Check sheet for the modelled part. Datum: model origin and axes. Units: mm. Face numbers are marked on the shaded views. A direction names the side the tool comes from. Coordinates: 2 decimals unless noted, no trailing zeros. Loops run counter-clockwise (first coordinate to the right, second up) from the corner with the lowest first, then second, coordinate; pieces in that order, holes last. Notation, with made-up numbers: (-7.75, 42) -> (20.25, 42) arc R17 cw to (20.25, 50) -> close; hole circle Ø5 at (40, 70.25). An arc over 180 degrees is marked (long way). Use CSV: the item, a comma, the result in double quotes. Start each with the question number.
1. Sectioned sample at D-D, the plane x = -35. Record the cut outline in (y, z), and give its area (3 significant figures).
2. Sectioned sample at A-A, the plane y = 54. Record the cut outline in (x, z).
3. Gauge pin test, flat ends, axial feed: pin 1 (1 mm diameter, centred on x = -18, z = -6, fed in from -Y); pin 2 (8 mm diameter, centred on x = 45.5, z = 3, fed in from +Y); pin 3 (2 mm diameter, centred on y = 45, z = -2.5, fed in from -X); pin 4 (2 mm diameter, centred on x = -7, z = 2, fed in from -Y). Record the tip position at first contact, or that the pin passes through.
4. Release check for a two-part mould opening along X. For the marked faces 1, 2, 3 and 4 record: pulls with the +X half, pulls with the -X half, needs draft (parallel to the pull), parting line crosses it, or undercut.
5. Set-up check for the marked faces 5, 6 and 7: record each of +Z, -Z, +X, -X, +Y, -Y from which the full face is reachable in a straight line by a thin tool's end or side.
6. Sectioned sample at B-B, the plane x = 0. Record the cut outline in (y, z).
7. Thickness scan on L1, parallel to X at y = 54, z = 5; L2, parallel to Y at x = -50, z = 7.5; L3, parallel to Y at x = 0, z = -2. Record the ranges inside material, lowest first.
8. Sectioned sample at C-C, the plane z = 8. Record the cut outline in (x, y).
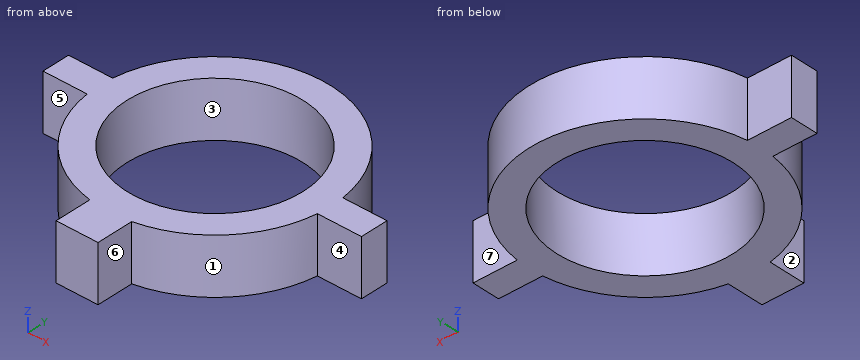
Autodesk Inventor part; units mm, degrees
ref_plane "YZ Plane" through (0, 0, 0) normal (1, 0, 0) x (0, 1, 0)
ref_plane "XZ Plane" through (0, 0, 0) normal (0, 1, 0) x (-1, 0, 0)
ref_plane "XY Plane" through (0, 0, 0) normal (0, 0, 1) x (1, 0, 0)
sketch "Sketch1" plane through (0, 0, 0) normal (0, 0, 1) x (1, 0, 0)
  circle A0 centre (0, 54) radius 31.5
  circle A1 centre (0, 54) radius 41.5
  line L0 (57, 49) -> (-57, 49)
  line L1 (-57, 49) -> (-57, 59)
  line L2 (-57, 59) -> (57, 59)
  line L3 (57, 59) -> (57, 49)
  line L4 (57, 49) -> (-57, 59) construction
  line L5 (-57, 49) -> (57, 59) construction
  line L6 (-7.5, 0) -> (7.5, 0)
  line L7 (7.5, 0) -> (7.5, 22.5)
  line L8 (7.5, 22.5) -> (-7.5, 22.5) construction
  line L9 (-7.5, 22.5) -> (-7.5, 0)
  point P0 (0, 0)
  point P1 (0, 0)
  point P2 (41.1977, 49)
  point P3 (41.1977, 59)
  point P4 (-41.1977, 59)
  point P5 (-41.1977, 49)
  point P6 (-7.5, 13.1833)
  point P7 (7.5, 13.1833)
  dimension "d0" = 54
  dimension "d2" = 10
  dimension "d3" = 63
  dimension "d4" = 10
  dimension "d5" = 114
  dimension "d6" = 15
extrude "Extrusion1" add sketch "Sketch1" along normal mid plane 20 contours A0 L2 A1 L0 | A0 L2 A1 | L0 A1 A0 | A0 L0 A1 L2 | L2 L3 L0 A1 | A1 L0 L1 L2 | L7 L6 L9 A1
equation "\"d4\" = d2"
properties part number "Pipe clamp bracket"
Completed:
1,outline,"(31.7, -10) -> (76.3, -10) -> (76.3, 10) -> (31.7, 10) -> close"
1,area,"892 mm²"
2,outline,"(-57, -10) -> (-31.5, -10) -> (-31.5, 10) -> (-57, 10) -> close; (31.5, -10) -> (57, -10) -> (57, 10) -> (31.5, 10) -> close"
3,pin 1,"y = 16.37"
3,pin 2,"y = 59"
3,pin 3,"x = -40.72"
3,pin 4,"y = 0"
4,face 1,"pulls with the +X half"
4,face 2,"pulls with the -X half"
4,face 3,"undercut"
4,face 4,"needs draft"
5,face 5,"+Z, -Z, -X, -Y"
5,face 6,"+Z, -Z, +X, -Y"
5,face 7,"+Z, -Z, +X, +Y"
6,outline,"(0, -10) -> (22.5, -10) -> (22.5, 10) -> (0, 10) -> close; (85.5, -10) -> (95.5, -10) -> (95.5, 10) -> (85.5, 10) -> close"
7,L1,"-57 to -31.5, 31.5 to 57"
7,L2,"49 to 59"
7,L3,"0 to 22.5, 85.5 to 95.5"
8,outline,"(-57, 49) -> (-41.2, 49) arc R41.5 ccw to (-7.5, 13.18) -> (-7.5, 0) -> (7.5, 0) -> (7.5, 13.18) arc R41.5 ccw to (41.2, 49) -> (57, 49) -> (57, 59) -> (41.2, 59) arc R41.5 ccw to (-41.2, 59) -> (-57, 59) -> close; hole circle Ø63 at (0, 54)"
